```python
from build123d import *

# Parameters (mm, degrees)
SKETCH1_R           = 1.5
SKETCH1_R_2         = 3
BOSS_EXTRUDE3_DEPTH = 4


with BuildPart() as part:
    # Sketch1 → Boss-Extrude3 (new body)
    with BuildSketch(Plane.XY):
        with BuildLine():
            Line((-200.98277671, 120.578395112), (-198.686273407, 120.032535791))
            ThreePointArc((-198.686273407, 120.032535791), (-190.744400987, 115.221467643), (-184.584385258, 108.273524028))
            ThreePointArc((-184.584385258, 108.273524028), (-181.272141891, 105.819229993), (-177.439106824, 107.336582128))
            ThreePointArc((-177.439106824, 107.336582128), (-172.13122346, 106.059599202), (-167.370398947, 103.387734467))
            Line((-167.370398947, 103.387734467), (-109.095690378, 45.714454225))
            Line((-109.095690378, 45.714454225), (-102.024771817, 45.714454225))
            Line((-102.024771817, 45.714454225), (-102.007026705, 52.767627674))
            Line((-102.007026705, 52.767627674), (-160.345422779, 110.504595422))
            ThreePointArc((-160.345422779, 110.504595422), (-163.078925024, 115.23029925), (-164.424771817, 120.521141112))
            ThreePointArc((-164.424771817, 120.521141112), (-162.39977496, 124.16226761), (-164.46612922, 127.780083873))
            ThreePointArc((-164.46612922, 127.780083873), (-171.220620663, 134.151626828), (-175.784254213, 142.238218389))
            Line((-175.784254213, 142.238218389), (-176.812194105, 147.245164825))
            ThreePointArc((-176.812194105, 147.245164825), (-179.718163472, 150.336336453), (-182.8093351, 147.430367085))
            Line((-182.8093351, 147.430367085), (-184.649305769, 140.159568784))
            ThreePointArc((-184.649305769, 140.159568784), (-187.814666362, 133.438140211), (-193.944387613, 129.240089815))
            Line((-193.944387613, 129.240089815), (-201.286490927, 127.709234194))
            ThreePointArc((-201.286490927, 127.709234194), (-202.714852362, 127.426883631), (-204.148777392, 127.174302472))
            ThreePointArc((-204.148777392, 127.174302472), (-206.658919771, 124.247833074), (-204.214354736, 121.266367045))
            ThreePointArc((-204.214354736, 121.266367045), (-202.594506126, 120.941450032), (-200.98277671, 120.578395112))
        make_face()
        with Locations((-117.274771817, 60.964454225)):
            Circle(SKETCH1_R, mode=Mode.SUBTRACT)
        with Locations((-180.524771817, 124.214454225)):
            Circle(SKETCH1_R_2, mode=Mode.SUBTRACT)
        with Locations((-124.382381975, 67.998789861)):
            Circle(SKETCH1_R, mode=Mode.SUBTRACT)
        with BuildLine():
            Line((-182.024547822, 132.114454225), (-182.024547822, 135.348786972))
            ThreePointArc((-182.024547822, 135.348786972), (-180.524727129, 136.848607665), (-179.024906436, 135.348786972))
            Line((-179.024906436, 135.348786972), (-179.024906436, 132.114454225))
            ThreePointArc((-179.024906436, 132.114454225), (-180.524727129, 130.614633532), (-182.024547822, 132.114454225))
        make_face(mode=Mode.SUBTRACT)
        with BuildLine():
            Line((-182.024547822, 116.314454225), (-182.024547822, 113.080121478))
            ThreePointArc((-182.024547822, 113.080121478), (-180.524727129, 111.580300785), (-179.024906436, 113.080121478))
            Line((-179.024906436, 113.080121478), (-179.024906436, 116.314454225))
            ThreePointArc((-179.024906436, 116.314454225), (-180.524727129, 117.814274918), (-182.024547822, 116.314454225))
        make_face(mode=Mode.SUBTRACT)
        with BuildLine():
            Line((-172.624771818, 125.71423023), (-169.39043907, 125.71423023))
            ThreePointArc((-169.39043907, 125.71423023), (-167.890618373, 124.214409533), (-169.39043907, 122.714588836))
            Line((-169.39043907, 122.714588836), (-172.624771818, 122.714588836))
            ThreePointArc((-172.624771818, 122.714588836), (-174.124592515, 124.214409533), (-172.624771818, 125.71423023))
        make_face(mode=Mode.SUBTRACT)
        with BuildLine():
            Line((-188.424754849, 125.714319606), (-191.659087596, 125.714356198))
            ThreePointArc((-191.659087596, 125.714356198), (-193.158925261, 124.214552469), (-191.659121532, 122.714714804))
            Line((-191.659121532, 122.714714804), (-188.424788785, 122.714678212))
            ThreePointArc((-188.424788785, 122.714678212), (-186.92495112, 124.214481941), (-188.424754849, 125.714319606))
        make_face(mode=Mode.SUBTRACT)
    extrude(amount=BOSS_EXTRUDE3_DEPTH)


solid = part.part
```
Model file for the job. Use its own axes, mm. A direction names the side the tool comes from. Coordinates: 2 decimals unless noted, no trailing zeros. Order: outer loops, then holes, each group sorted by start corner. A loop starts at its lowest first (then second) coordinate and runs counter-clockwise, first axis right, second up. Notation, with made-up numbers: (71.5, -11) - (78.5, -11) arc R18 ccw to (78.5, 2) - close; hole circle Ø6 at (10, 18). An arc over 180 degrees is marked (long way). Return JSON: item names as keys, results as strings. Group by question number.
1) Saw through at A-A, the plane z = 1.75. Count the separate pieces of the cut face and the enclosed holes in it, plus the area to 3 significant figures.
2) Saw through at B-B, the plane x = -157. Write the cut outline in (y, z), plus the area to 3 significant figures.
3) Flat gauge pins, fed straight in: P1, Ø1, axis at x = -158.5, y = 92.5, coming from the -Z side; P2, Ø1, axis at x = -170.5, z = 1.5, coming from the +Y side; P3, Ø1, axis at y = 114.5, z = 1, coming from the -X side; P4, Ø1.6, axis at x = -189.5, z = 2, coming from the -Y side. Where does each tip first touch, or does it go through?
4) Tool access for faces 1 (the flat face through (-171, 122.715, 2)), 2 (the cylindrical face through (-181.332, 105.827, 1.972)): list every direction of +Z, -Z, +X, -X, +Y, -Y with a clear straight run to the whole face (end or side of a thin tool).
5) Probe line 1 (X direction, y = 135, z = 1.95); line 2 (X direction, y = 68.5, z = 3.4); line 3 (Y direction, x = -181, z = 0.2). List the from-to ranges inside material, lowest first. Write a range as from..to.
6) Saw through at C-C, the plane y = 92.5. Write the cut outline in (x, z), plus the area to 3 significant figures.
7) Mould opens along Y. For faces 3 (the flat face through (-182.025, 115, 2)), 4 (the cylindrical face through (-202.69, 127.43, 1.97)), 5 (the cylindrical face through (-202.617, 120.946, 1.972)) say: released by +Y, released by -Y, zero draft, split by the parting line, or undercut.
Values found:
{
 "1": {"separate pieces": "1", "enclosed holes": "7", "area": "1,730 mm²"},
 "2": {"outline": "(93.12, 0) - (107.19, 0) - (107.19, 4) - (93.12, 4) - close", "area": "56.3 mm²"},
 "3": {"P1": "passes through", "P2": "stops at y = 133.87", "P3": "stops at x = -190.48", "P4": "stops at y = 113.36"},
 "4": {"face 1": "+Z, -Z", "face 2": "+Z, -Z, -Y"},
 "5": {"line 1": "x = -186.66..-182.02, -179.02..-171.86", "line 2": "x = -132.12..-125.8, -122.97..-117.9", "line 3": "y = 105.79..111.66, 117.74..121.25, 127.18..130.69, 136.77..150.09"},
 "6": {"outline": "(-156.37, 0) - (-142.15, 0) - (-142.15, 4) - (-156.37, 4) - close", "area": "56.9 mm²"},
 "7": {"face 3": "undercut", "face 4": "released by +Y", "face 5": "released by -Y"}
}
